Part model, mm, in its own coordinate system. Face numbers are marked on the shaded views. Round coordinates to 2 decimals unless told otherwise and drop trailing zeros. Write each loop counter-clockwise with the first axis right and the second up, starting at its lowest first coordinate (ties: lowest second). Pieces come first, ordered by that corner, then holes.
from build123d import *

# Parameters (mm, degrees)
SKETCH2_W           = 25
SKETCH2_H           = 10.7
BOSS_EXTRUDE1_DEPTH = 3.2
SKETCH3_R           = 1.5
CUT_EXTRUDE2_DEPTH  = 3.2
SKETCH4_W           = 0.284935898
SKETCH4_H           = 3.175
CUT_EXTRUDE3_DEPTH  = 0.254


with BuildPart() as part:
    # Sketch2 → Boss-Extrude1 (new body)
    with BuildSketch(Plane.XY):
        with Locations((0.072254335, -5.35)):
            Rectangle(SKETCH2_W, SKETCH2_H)
    extrude(amount=BOSS_EXTRUDE1_DEPTH)

    # Sketch3 → Cut-Extrude2 (cut)
    with BuildSketch(Plane.XY.offset(3.2)):
        with Locations((-10.814046376, -5.35)):
            Circle(SKETCH3_R)
        with Locations(Location((10.958555047, -5.35, 0), (0, 0, 180))):
            Circle(SKETCH3_R)
    extrude(amount=-CUT_EXTRUDE2_DEPTH, mode=Mode.SUBTRACT)

    # Sketch4 → Cut-Extrude3 (cut)
    # profile 1 of 5: a face of its own
    with BuildSketch(Plane.XY.offset(3.2)):
        Polygon((-5.243533556, -2.175), (-4.958597658, -2.175), (-4.958597658, -5.024358974), (-3.737443812, -5.024358974), (-3.737443812, -5.35), (-5.243533556, -5.35), align=None)
    # profile 2 of 5: a face of its own
    with BuildSketch(Plane.XY.offset(3.2)):
        with Locations((-3.065809197, -3.7625)):
            Rectangle(SKETCH4_W, SKETCH4_H)
    # profile 3 of 5: a face of its own
    with BuildSketch(Plane.XY.offset(3.2)):
        with BuildLine():
            Line((-2.109238684, -5.35), (-2.109238684, -2.175))
            Line((-2.109238684, -2.175), (-1.468132915, -2.175))
            add(Edge.make_bspline(
                [(-1.468132915, -2.175), (-1.412371761, -2.175401474), (-1.304641503, -2.17617712), (-1.148964497, -2.181095097), (-1.004924941, -2.189795019), (-0.872996561, -2.202467375), (-0.752817176, -2.218027627), (-0.644723296, -2.237531565), (-0.548155995, -2.260562263), (-0.48876586, -2.280197778), (-0.460680992, -2.289483173)],
                knots=[0, 0, 0, 0, 1.314313732, 2.53924729, 3.670748893, 4.714932338, 5.66265055, 6.526160246, 7.303039223, 8, 8, 8, 8], degree=3))
            add(Edge.make_bspline(
                [(-0.460680992, -2.289483173), (-0.423946478, -2.303481027), (-0.351310468, -2.331159311), (-0.247889721, -2.383371099), (-0.150530285, -2.442528698), (-0.05871006, -2.508710088), (0.025473546, -2.583789176), (0.105309281, -2.664576675), (0.177531209, -2.754010383), (0.243669449, -2.850235551), (0.303301083, -2.952118627), (0.355134462, -3.059465476), (0.398182013, -3.171730943), (0.433917297, -3.288602827), (0.462080869, -3.410338113), (0.481295908, -3.537078548), (0.493969591, -3.668323242), (0.495243266, -3.757381505), (0.495889521, -3.802569111)],
                knots=[0, 0, 0, 0, 0.984719456, 1.947108742, 2.898477687, 3.838006223, 4.779231079, 5.722358779, 6.681677486, 7.655904652, 8.64651281, 9.637519902, 10.640069247, 11.656948941, 12.698408672, 13.768548281, 14.867775369, 16, 16, 16, 16], degree=3))
            add(Edge.make_bspline(
                [(0.495889521, -3.802569111), (0.495318958, -3.841813234), (0.494194603, -3.919147878), (0.484098724, -4.033122119), (0.46942449, -4.143715145), (0.446705825, -4.250400316), (0.419126402, -4.354112342), (0.383780351, -4.453745878), (0.343289579, -4.550214905), (0.296072904, -4.642215044), (0.244237505, -4.729376388), (0.188609923, -4.811541332), (0.129249492, -4.887537426), (0.065590168, -4.95759481), (-0.001545403, -5.02160787), (-0.07259676, -5.080111341), (-0.147747242, -5.131960502), (-0.226660255, -5.179192807), (-0.311637886, -5.220395558), (-0.404289708, -5.255257067), (-0.505010848, -5.284146497), (-0.61355408, -5.308250095), (-0.730106949, -5.327370219), (-0.854783725, -5.340184875), (-0.987392852, -5.34885075), (-1.078451186, -5.349609478), (-1.125319413, -5.35)],
                knots=[0, 0, 0, 0, 1.105936401, 2.179363191, 3.223086493, 4.248585256, 5.251745608, 6.245858792, 7.225916811, 8.198733463, 9.158002045, 10.082870192, 10.993790845, 11.873723703, 12.748670949, 13.606408763, 14.465103618, 15.319838547, 16.196477973, 17.123216899, 18.106603292, 19.147568657, 20.255746949, 21.433717677, 22.679120308, 24, 24, 24, 24], degree=3))
            Line((-1.125319413, -5.35), (-2.109238684, -5.35))
        make_face()
        with BuildLine():
            Line((-1.824302787, -5.024358974), (-1.459864686, -5.024358974))
            add(Edge.make_bspline(
                [(-1.459864686, -5.024358974), (-1.407496806, -5.024133916), (-1.306774196, -5.023701045), (-1.161941585, -5.019902653), (-1.029608132, -5.013696039), (-0.909755049, -5.005010075), (-0.802450005, -4.993517832), (-0.707468746, -4.980704527), (-0.625122619, -4.964741125), (-0.575293773, -4.950271326), (-0.55226753, -4.943584736)],
                knots=[0, 0, 0, 0, 1.375205317, 2.645023457, 3.804390687, 4.853969522, 5.800190428, 6.637939096, 7.370582563, 8, 8, 8, 8], degree=3))
            add(Edge.make_bspline(
                [(-0.55226753, -4.943584736), (-0.523285802, -4.933377965), (-0.466014573, -4.913208212), (-0.383572445, -4.876416619), (-0.306685734, -4.832835599), (-0.234014497, -4.784392108), (-0.166589602, -4.72937752), (-0.103612011, -4.668988123), (-0.04520852, -4.602916577), (0.00801746, -4.531244888), (0.055649992, -4.454419144), (0.096898893, -4.373194631), (0.133049926, -4.28846131), (0.161424078, -4.198918002), (0.183663215, -4.105365213), (0.199415467, -4.007796363), (0.209225967, -3.906229671), (0.210370281, -3.837148816), (0.210953624, -3.801933093)],
                knots=[0, 0, 0, 0, 0.998632004, 1.973411704, 2.929992603, 3.868527914, 4.809262121, 5.754881198, 6.702106254, 7.672490631, 8.653608572, 9.636854334, 10.631411391, 11.644891563, 12.686317036, 13.754757253, 14.855430412, 16, 16, 16, 16], degree=3))
            add(Edge.make_bspline(
                [(0.210953624, -3.801933093), (0.210487999, -3.764800579), (0.209573274, -3.691853426), (0.198075864, -3.584819009), (0.181274167, -3.481875848), (0.156977538, -3.383017056), (0.126015955, -3.288049765), (0.08737653, -3.19749921), (0.043228954, -3.110409079), (-0.009297645, -3.028789475), (-0.066824647, -2.951597869), (-0.130667438, -2.880881624), (-0.199811715, -2.816479652), (-0.273503329, -2.75738899), (-0.353819126, -2.705986941), (-0.438867117, -2.66000688), (-0.529894976, -2.620985322), (-0.593225064, -2.600230925), (-0.625409557, -2.589683494)],
                knots=[0, 0, 0, 0, 1.122418816, 2.205001699, 3.251619955, 4.274784885, 5.280384055, 6.268708349, 7.249350384, 8.229342522, 9.199999885, 10.157847722, 11.105861043, 12.055065948, 13.010012805, 13.98527497, 14.976112212, 16, 16, 16, 16], degree=3))
            add(Edge.make_bspline(
                [(-0.625409557, -2.589683494), (-0.65203524, -2.582320734), (-0.708648747, -2.566665487), (-0.801031689, -2.549588185), (-0.905004004, -2.534525532), (-1.021027304, -2.521772882), (-1.148969335, -2.512622241), (-1.288928494, -2.505753977), (-1.440965279, -2.501121532), (-1.546359434, -2.500805204), (-1.601060599, -2.500641026)],
                knots=[0, 0, 0, 0, 0.674548936, 1.434276114, 2.292660221, 3.240891867, 4.284742987, 5.42552168, 6.663806718, 8, 8, 8, 8], degree=3))
            Line((-1.601060599, -2.500641026), (-1.824302787, -2.500641026))
            Line((-1.824302787, -2.500641026), (-1.824302787, -5.024358974))
        make_face(mode=Mode.SUBTRACT)
    # profile 4 of 5: a face of its own
    with BuildSketch(Plane.XY.offset(3.2)):
        Polygon((2.449735675, -2.175), (3.91512029, -5.35), (3.605379705, -5.35), (3.135998696, -4.332371795), (1.696690803, -4.332371795), (1.214589441, -5.35), (0.902940803, -5.35), (2.409030547, -2.175), align=None)
        Polygon((2.426203023, -2.79448117), (1.851879104, -4.006730769), (2.985898536, -4.006730769), align=None, mode=Mode.SUBTRACT)
    # profile 5 of 5: a face of its own
    with BuildSketch(Plane.XY.offset(3.2)):
        with BuildLine():
            Line((4.484992085, -2.175), (5.120373696, -2.175))
            add(Edge.make_bspline(
                [(5.120373696, -2.175), (5.162774577, -2.175141139), (5.244188965, -2.175412141), (5.360823289, -2.176923226), (5.466802155, -2.181254248), (5.562070152, -2.18498132), (5.646625532, -2.191777582), (5.720727574, -2.198273311), (5.784034986, -2.206776561), (5.822358008, -2.214673623), (5.839709633, -2.218249199)],
                knots=[0, 0, 0, 0, 1.410062039, 2.707475311, 3.878576406, 4.937260626, 5.877586885, 6.699081471, 7.410979367, 8, 8, 8, 8], degree=3))
            add(Edge.make_bspline(
                [(5.839709633, -2.218249199), (5.862938499, -2.223988479), (5.908900697, -2.235344604), (5.975076828, -2.259347242), (6.038136251, -2.287123616), (6.09781702, -2.319747848), (6.153820202, -2.357462112), (6.206723241, -2.399615338), (6.256766197, -2.445976874), (6.301925247, -2.497715623), (6.344505673, -2.551995886), (6.380418213, -2.610691437), (6.411375805, -2.672070108), (6.436023345, -2.736756123), (6.455869793, -2.804122159), (6.469863596, -2.874778424), (6.478255744, -2.948403023), (6.479110142, -2.998620555), (6.479543367, -3.024083534)],
                knots=[0, 0, 0, 0, 1.027469482, 2.033020251, 3.019912614, 3.986113645, 4.951240523, 5.91722682, 6.890402269, 7.87763091, 8.8651537, 9.85103654, 10.82876324, 11.815024772, 12.821070561, 13.842952187, 14.906261191, 16, 16, 16, 16], degree=3))
            add(Edge.make_bspline(
                [(6.479543367, -3.024083534), (6.478210776, -3.066388236), (6.475610546, -3.148935667), (6.451367059, -3.268733752), (6.411655502, -3.380484059), (6.356933661, -3.48404588), (6.287247422, -3.577400537), (6.203495647, -3.659397593), (6.105631614, -3.728013799), (6.014527877, -3.775595987), (5.934051425, -3.806069554), (5.867799777, -3.827511108), (5.795530447, -3.844077319), (5.717935865, -3.858918296), (5.634693121, -3.870123047), (5.546001728, -3.878329601), (5.451798433, -3.883458631), (5.387083706, -3.884222449), (5.353792165, -3.884615385)],
                knots=[0, 0, 0, 0, 1.260483769, 2.459530307, 3.627416485, 4.787058657, 5.939039949, 7.08810263, 8.267026773, 9.491475466, 10.141966685, 10.831826277, 11.566392101, 12.351337768, 13.187381173, 14.07005841, 15.007169909, 16, 16, 16, 16], degree=3))
            Line((5.353792165, -3.884615385), (6.520248495, -5.35))
            Line((6.520248495, -5.35), (6.167894729, -5.35))
            Line((6.167894729, -5.35), (5.001438399, -3.884615385))
            Line((5.001438399, -3.884615385), (4.769927983, -3.884615385))
            Line((4.769927983, -3.884615385), (4.769927983, -5.35))
            Line((4.769927983, -5.35), (4.484992085, -5.35))
            Line((4.484992085, -5.35), (4.484992085, -2.175))
        make_face()
        with BuildLine():
            Line((4.769927983, -2.500641026), (4.769927983, -3.558974359))
            Line((4.769927983, -3.558974359), (5.351248095, -3.563426482))
            add(Edge.make_bspline(
                [(5.351248095, -3.563426482), (5.378389844, -3.56343849), (5.430998286, -3.563461764), (5.507108174, -3.559838838), (5.577974276, -3.5557174), (5.643325529, -3.54941335), (5.70319113, -3.541288914), (5.757541155, -3.531126207), (5.806464323, -3.519286121), (5.863522283, -3.500960361), (5.927236851, -3.47192633), (5.996480389, -3.429684771), (6.055446796, -3.376554212), (6.105265142, -3.31579972), (6.145296841, -3.249001123), (6.173519919, -3.176959131), (6.191429134, -3.101492467), (6.193541458, -3.049623755), (6.19460747, -3.023447516)],
                knots=[0, 0, 0, 0, 1.146690395, 2.22261258, 3.21895312, 4.145990853, 4.996080663, 5.770904154, 6.481378293, 7.121626537, 8.300444488, 9.431385265, 10.535395872, 11.636531494, 12.74115979, 13.810798291, 14.895190096, 16, 16, 16, 16], degree=3))
            add(Edge.make_bspline(
                [(6.19460747, -3.023447516), (6.193516974, -2.997914553), (6.19135601, -2.947317536), (6.173713199, -2.87324396), (6.143877831, -2.803333227), (6.10367123, -2.73786973), (6.054686282, -2.67844667), (5.99724798, -2.627603895), (5.932926839, -2.585649024), (5.872809395, -2.558838978), (5.819075502, -2.542401683), (5.772421453, -2.530834556), (5.719706041, -2.521541359), (5.660673304, -2.514095475), (5.595575253, -2.507695633), (5.524082734, -2.503385091), (5.446670083, -2.500832514), (5.393015367, -2.500706341), (5.365240483, -2.500641026)],
                knots=[0, 0, 0, 0, 1.101028733, 2.181837193, 3.264309656, 4.369019818, 5.486613113, 6.575447106, 7.666700264, 8.788928104, 9.402425223, 10.0903467, 10.862060571, 11.710948788, 12.657782767, 13.684531032, 14.801375019, 16, 16, 16, 16], degree=3))
            Line((5.365240483, -2.500641026), (4.769927983, -2.500641026))
        make_face(mode=Mode.SUBTRACT)
    extrude(amount=-CUT_EXTRUDE3_DEPTH, mode=Mode.SUBTRACT)


solid = part.part
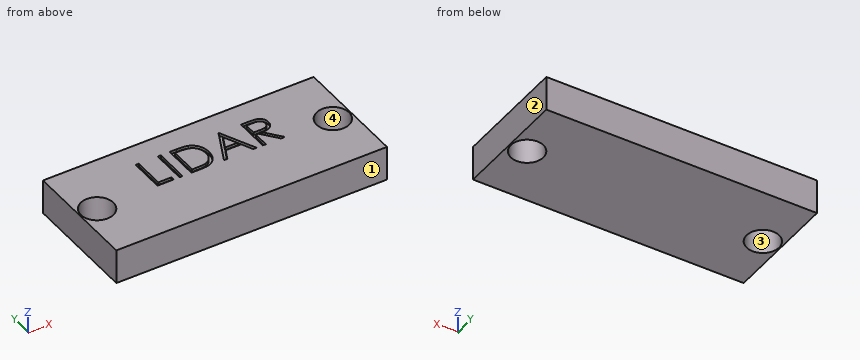
Q1. Drop a flat-ended pin along its axis: P1, Ø1, axis at x = 3.5, y = -9, coming from the -Z side. Give the stop position or say it passes through.
Q2. Two-plate mould, pull along X, no slides. Class the marked faces 1, 2, 3 and 4: released by +X, released by -X, zero draft, split by the parting line, or undercut.
Q3. Wall check: line 1 (X direction, y = -6.5, z = 3); line 2 (X direction, y = -4.75, z = 2.75); line 3 (Y direction, x = 11, z = 2). Give the ranges that are in metal, low to high.
Q4. Saw through at B-B, the plane y = -6.5. Write the cut outline in (x, z), and give its area (3 significant figures).
Q5. Saw through at A-A, the plane z = 1.25. Write the cut outline in (x, y), and give its area (3 significant figures).
Computed:
1. P1: stops at z = 0
2. face 1: zero draft
2. face 2: released by +X
2. face 3: undercut
2. face 4: undercut
3. line 1: x = -12.43 to -11.78, -9.85 to 10, 11.92 to 12.57
3. line 2: x = -12.43 to -12.19, -9.44 to 9.58, 12.33 to 12.57
3. line 3: y = -10.7 to -6.85, -3.85 to 0
4. outline: (-12.43, 0) - (-11.78, 0) - (-11.78, 3.2) - (-12.43, 3.2) - close; (-9.85, 0) - (10, 0) - (10, 3.2) - (-9.85, 3.2) - close; (11.92, 0) - (12.57, 0) - (12.57, 3.2) - (11.92, 3.2) - close
4. area: 67.7 mm2
5. outline: (-12.43, -10.7) - (12.57, -10.7) - (12.57, 0) - (-12.43, 0) - close; hole circle Ø3 at (-10.81, -5.35); hole circle Ø3 at (10.96, -5.35)
5. area: 253 mm2
